Here's how the part is built. I have some questions about the finished solid (model axes, mm). A direction names the side the tool comes from. Round coordinates to 2 decimals unless told otherwise and drop trailing zeros. Write each loop counter-clockwise with the first axis right and the second up, starting at its lowest first coordinate (ties: lowest second). Pieces come first, ordered by that corner, then holes. Notation, with made-up numbers: (0, -34.75) -> (36, -34.75) arc R10 cw to (36, -26.75) -> close; hole circle Ø4 at (26.5, 28). An arc over 180 degrees is marked (long way). Answer as CSV lines item,"result".
Autodesk Fusion 360 part; units mm, degrees
sketch "Esquisse1" plane through (0, 0, 0) normal (0, 0, 1) x (1, 0, 0)
  circle A0 centre (0, 0) radius 17
  circle A1 centre (0, 0) radius 6.2
  dimension "d1" = 34
  dimension "d2" = 12.4
extrude "Extrusion1" add sketch "Esquisse1" along normal blind 22.2 contours A0 | A1
extrude "Extrusion2" cut sketch "Esquisse1" along normal blind 18.5 contours A1
hole "Perçage1" at (0, -17, 8) direction (0, 1, 0) diameter 5.5 depth 17 tip angle 180
ref_plane "Plan de construction1" through (0, -13, 0) normal (0, 1, 0) x (0, 0, 1)
sketch "Esquisse2" plane through (0, -13, 0) normal (0, 1, 0) x (1, 0, 0)
  line L0 (-4.1, 0) -> (4.1, 0)
  line L1 (4.1, 0) -> (4.1, -8)
  line L2 (-4.1, -8) -> (-4.1, 0)
  line L3 (-4.1, -10.3671) -> (0, -12.7343)
  line L4 (0, -12.7343) -> (4.1, -10.3671)
  line L5 (-4.1, -10.3671) -> (-4.1, -8)
  line L6 (4.1, -10.3671) -> (4.1, -8)
  point P0 (0, -8)
  dimension "d12" = 8.2
  dimension "d13" = 4.1
  dimension "d14" = 8
extrude "Extrusion3" cut sketch "Esquisse2" along normal blind 4.9
extrude "Extrusion4" add 1 faces at (1.6321, -3.8543, 22.2) along direction (0, 0, 1) blind 20
sketch "Esquisse5" plane through (0, 0, 42.2) normal (0, 0, 1) x (-1, 0, 0)
  circle A0 centre (0, 0) radius 17
  line L0 (8.5, 5.1) -> (-8.5, 5.1)
  line L1 (-8.5, 5.1) -> (-8.5, 1.7)
  line L2 (-8.5, 1.7) -> (8.5, 1.7)
  line L3 (8.5, 1.7) -> (8.5, 5.1)
  line L4 (11.5333, 0) -> (-9, 0) construction
  line L5 (-8.5, -1.7) -> (8.5, -1.7)
  line L6 (8.5, -1.7) -> (8.5, -5.1)
  line L7 (8.5, -5.1) -> (-8.5, -5.1)
  line L8 (-8.5, -5.1) -> (-8.5, -1.7)
  dimension "d20" = 17
  dimension "d21" = 3.4
  dimension "d22" = 8.5
  dimension "d23" = 1.7
extrude "Extrusion5" cut sketch "Esquisse5" against normal blind 16.5 contours L0 L1 L2 L3 | L5 L6 L7 L8
hole "Perçage2" at (0, -17, 34.2) direction (0, 1, 0) diameter 5.5 depth 41 tip angle 180 counterbore diameter 9 counterbore depth 7
sketch "Esquisse6" plane through (0, 0, 0) normal (0, 1, 0) x (1, 0, 0)
ref_plane "Plan de construction2" through (0, 17, 0) normal (0, 1, 0) x (0, 0, 1)
sketch "Esquisse7" plane through (0, 17, 0) normal (0, 1, 0) x (1, 0, 0)
  line L0 (0.2093, -36.942) -> (6.8092, -36.4383) construction
  circle A0 centre (0, -34.2) radius 2.75
  line L1 (0.2093, -36.942) -> (0, -34.2) construction
  line L2 (-4.1594, -31.7062) -> (-4.2394, -36.5552)
  line L3 (-4.2394, -36.5552) -> (-0.08, -39.0491)
  line L4 (-0.08, -39.0491) -> (4.1594, -36.6938)
  line L5 (4.1594, -36.6938) -> (4.2394, -31.8448)
  line L6 (4.2394, -31.8448) -> (0.08, -29.3509)
  line L7 (0.08, -29.3509) -> (-4.1594, -31.7062)
  point P0 (0, -34.2)
  dimension "d33" = 4.2
extrude "Extrusion6" cut sketch "Esquisse7" against normal blind 5
chamfer "Chanfrein1" distance 0.5 angle 45 8 edges at (0, 1.7, 42.2) (8.5, 3.4, 42.2) (0, 5.1, 42.2) (-8.5, 3.4, 42.2) (0, -1.7, 42.2) (-8.5, -3.4, 42.2) (0, -5.1, 42.2) (8.5, -3.4, 42.2)
chamfer "Chanfrein2" distance 1 angle 45 2 edges at (4.5, -16.3936, 34.2) (-4.5, -16.3936, 34.2)
chamfer "Chanfrein3" distance 1 angle 45 6 edges at (2.1763, 16.8601, 30.6078) (4.1994, 16.4732, 34.2685) (2.056, 16.8752, 37.8624) (-2.1763, 16.8601, 37.7922) (-4.1994, 16.4732, 34.1315) (-2.056, 16.8752, 30.5376)
fillet "Congé1" radius 1 1 edges at (-15.8496, -6.1475, 42.2)
equation "d13 = d12 / 2"
equation "d22 = d20 / 2"
equation "d23 = ( 3.4 / 2 ) * 1 mm"
1. Suppose I cut it at B-B on z = 8. Please give me the cut outline in (x, y), and give its area (3 significant figures).
Numbers:
outline,"(-4.1, -13) -> (-4.1, -8.1) -> (-2.75, -8.1) -> (-2.75, -5.56) arc R6.2 cw (long way) to (2.75, -5.56) -> (2.75, -8.1) -> (4.1, -8.1) -> (4.1, -13) -> (2.75, -13) -> (2.75, -16.78) arc R17 ccw (long way) to (-2.75, -16.78) -> (-2.75, -13) -> close"
area,"714 mm^2"
2. If I drill on line 1 (Y direction, x = -1, z = 31); line 2 (Z direction, x = 0, y = -15.55); line 3 (Z direction, x = 0, y = 8.25), over which ranges is the centre line in solid material (lowest first)?
Numbers:
line 1,"y = -10 to -5.1, -1.7 to 1.7, 5.1 to 12"
line 2,"z = 0 to 5.25, 10.75 to 29.7, 38.7 to 42.2"
line 3,"z = 0 to 31.45, 36.95 to 42.2"
3. For pin 1 Ø1.5 at (y, z) = (-6.5, 32) entering from +X; pin 2 Ø5.5 at (y, z) = (-9.5, 5) entering from +X; pin 3 Ø4.5 at (x, z) = (-1.5, 34) entering from -Y, each with a flat end and sliding along its axis, tell me the tip position at first contact or that it passes through.
Numbers:
pin 1,"stops at x = 16"
pin 2,"stops at x = 15.6"
pin 3,"stops at y = -10"
4. Suppose I cut it at A-A on y = 0. Please give me the cut outline in (x, z).
Numbers:
outline,"(-17, 0) -> (-6.2, 0) -> (-6.2, 18.5) -> (6.2, 18.5) -> (6.2, 0) -> (17, 0) -> (17, 41.2) arc R1 ccw to (16, 42.2) -> (-16, 42.2) arc R1 ccw to (-17, 41.2) -> close; hole circle Ø5.5 at (0, 34.2)"
5. If we mould it in two halves opening along X, with no side actions, what happens to faces 4 (the face through (7, 0, 0)), 5 (the face through (-0.198, -12.958, 38.696)), 6 (the face through (8, 15, 20))? For each: released by +X, released by -X, zero draft, split by the parting line, or undercut.
Numbers:
face 4,"zero draft"
face 5,"undercut"
face 6,"split by the parting line"
6. On a 3-axis mill with a long thin cutter (end or side, diameter ignored), from which of +Z, -Z, +X, -X, +Y, -Y can I reach the whole of each face in a straight line? I mean faces 1 (the face through (-4.1, -11, 5)), 2 (the face through (-2.01, 14.03, 30.51)), 3 (the face through (0, -3, 25.7)). Say none if no direction works.
Numbers:
face 1,"-Z"
face 2,"+Y"
face 3,"+Z"
